```python
from build123d import *

# Parameters (mm, degrees)
ENL_V_START             = -12
ENL_V_MAT_EXTRU_1_DEPTH = 12
ENL_V_START_2           = -3
ENL_V_MAT_EXTRU_2_DEPTH = 3
CHANFREIN1_SIZE         = 1
ENL_V_MAT_EXTRU_3_DEPTH = 3
ESQUISSE5_R             = 0.75
BOSS_EXTRU_1_DEPTH      = 0.5
CONG_1_R                = 0.5
ESQUISSE6_R             = 1.5
ENL_V_MAT_EXTRU_4_DEPTH = 5.5
CHANFREIN2_SIZE         = 1


with BuildPart() as part:
    # Esquisse1 → Révolution1 (revolve)
    with BuildSketch(Plane.XY):
        Polygon((0, 0), (0, 3), (17, 3), (17, 10), (20, 10), (20, 16), (60, 16), (60, 13.75), (100.5, 13.75), (100.5, 0), align=None)
    revolve(axis=Axis((100.5, 0, 0), (-1, 0, 0)))

    # Esquisse2 → Enlèv. mat.-Extru.1 (cut)
    with BuildSketch(Plane.ZY.offset(ENL_V_START)):
        with BuildLine():
            Line((-1.658312395, 2.5), (1.658312395, 2.5))
            ThreePointArc((1.658312395, 2.5), (0, 3), (-1.658312395, 2.5))
        make_face()
    extrude(amount=ENL_V_MAT_EXTRU_1_DEPTH, mode=Mode.SUBTRACT)

    # Esquisse3 → Enlèv. mat.-Extru.2 (cut)
    with BuildSketch(Plane.ZY.offset(-17).offset(ENL_V_START_2)):
        with BuildLine():
            ThreePointArc((-9, 4.358898944), (-10, 0), (-9, -4.358898944))
            Line((-9, -4.358898944), (-9, 4.358898944))
        make_face()
        with BuildLine():
            Line((9, 4.358898944), (9, -4.358898944))
            ThreePointArc((9, -4.358898944), (9.746794345, -2.236067977), (10, 0))
            ThreePointArc((10, 0), (9.746794345, 2.236067977), (9, 4.358898944))
        make_face()
    extrude(amount=ENL_V_MAT_EXTRU_2_DEPTH, mode=Mode.SUBTRACT)

    # Chanfrein1
    chanfrein1_edges = [part.edges().sort_by_distance(p)[0] for p in [
        (20, -16, 0),
    ]]
    chamfer(chanfrein1_edges, length=CHANFREIN1_SIZE)

    # Esquisse4 → Enlèv. mat.-Extru.3 (cut)
    with BuildSketch(Plane.ZY.offset(-20)):
        with BuildLine():
            Line((16, 1.5), (15, 1.5))
            ThreePointArc((15, 1.5), (13.5, 0), (15, -1.5))
            Line((15, -1.5), (16, -1.5))
            Line((16, -1.5), (16, 1.5))
        make_face()
        with BuildLine():
            Line((1.5, -16), (1.5, -15))
            ThreePointArc((1.5, -15), (0, -13.5), (-1.5, -15))
            Line((-1.5, -15), (-1.5, -16))
            Line((-1.5, -16), (1.5, -16))
        make_face()
        with BuildLine():
            Line((-16, -1.5), (-15, -1.5))
            ThreePointArc((-15, -1.5), (-13.5, 0), (-15, 1.5))
            Line((-15, 1.5), (-16, 1.5))
            Line((-16, 1.5), (-16, -1.5))
        make_face()
        with BuildLine():
            Line((-1.5, 16), (-1.5, 15))
            ThreePointArc((-1.5, 15), (0, 13.5), (1.5, 15))
            Line((1.5, 15), (1.5, 16))
            Line((1.5, 16), (-1.5, 16))
        make_face()
    extrude(amount=-ENL_V_MAT_EXTRU_3_DEPTH, mode=Mode.SUBTRACT)

    # Esquisse5 → Boss.-Extru.1 (add)
    with BuildSketch(Plane.ZY.offset(-23)):
        with Locations(Location((0, 15, 0), (0, 0, 270))):
            Circle(ESQUISSE5_R)
        with Locations(Location((15, 0, 0), (0, 0, 270))):
            Circle(ESQUISSE5_R)
        with Locations(Location((0, -15, 0), (0, 0, 270))):
            Circle(ESQUISSE5_R)
        with Locations(Location((-15, 0, 0), (0, 0, 270))):
            Circle(ESQUISSE5_R)
    extrude(amount=BOSS_EXTRU_1_DEPTH)

    # Congé1
    cong_1_edges = [part.edges().sort_by_distance(p)[0] for p in [
        (22.5, 15.75, 0),
        (22.5, 0.75, 15),
        (22.5, -14.25, 0),
        (22.5, 0.75, -15),
    ]]
    fillet(cong_1_edges, radius=CONG_1_R - 0.0001)  # a hair under: the kernel refuses the full size

    # Esquisse6 → Enlèv. mat.-Extru.4 (cut)
    with BuildSketch(Plane.ZY.offset(-20)):
        with Locations(Location((9.192388155, 9.192388155, 0), (0, 0, 270))):
            Circle(ESQUISSE6_R)
        with Locations(Location((9.192388155, -9.192388155, 0), (0, 0, 270))):
            Circle(ESQUISSE6_R)
        with Locations(Location((-9.192388155, -9.192388155, 0), (0, 0, 270))):
            Circle(ESQUISSE6_R)
        with Locations(Location((-9.192388155, 9.192388155, 0), (0, 0, 270))):
            Circle(ESQUISSE6_R)
    extrude(amount=-ENL_V_MAT_EXTRU_4_DEPTH, mode=Mode.SUBTRACT)

    # Chanfrein2
    chanfrein2_edges = [part.edges().sort_by_distance(p)[0] for p in [
        (100.5, -13.75, 0),
    ]]
    chamfer(chanfrein2_edges, length=CHANFREIN2_SIZE)


solid = part.part
```
Geometry check sheet. Reference: the model listing, model coordinates, mm. A direction names the side the tool comes from. Round coordinates to 2 decimals unless told otherwise and drop trailing zeros. Order: outer loops, then holes, each group sorted by start corner. A loop starts at its lowest first (then second) coordinate and runs counter-clockwise, first axis right, second up. Notation, with made-up numbers: (25.5, -39.75) - (33.5, -39.75) arc R25 cw to (33.5, -21.75) - close; hole circle Ø6 at (51, 27.25). An arc over 180 degrees is marked (long way). Use a Markdown table: item, result. Add a question column.
1) Set-up check for faces 1 (the conical face through (20.174, 10.625, 10.833)), 2 (the flat face through (0, 0, 0)), 3 (the cylindrical face through (19, -10, 0)), 4 (the cylindrical face through (80.026, -2.981, 13.423)), 5 (the flat face through (17, 2.4, -2.1)): record each of +Z, -Z, +X, -X, +Y, -Y from which the full face is reachable in a straight line by a thin tool's end or side.
2) Thickness scan on line 1 along X through (y, z) = (1.5, -10); line 2 along Y through (x, z) = (63.5, 2.5); line 3 along X through (y, z) = (-2, 5). Record the ranges inside material, lowest first.
3) Gauge pin test, flat ends, axial feed: P1, Ø2.5, axis at y = -10, z = 9, coming from the -X side; P2, Ø1.8, axis at y = -9.19, z = -9.19, coming from the -X side; P3, Ø0.9, axis at x = 18, y = -0.5, coming from the +Z side; P4, Ø5.5, axis at y = 2.5, z = -2, coming from the -X side. Record the tip position at first contact, or that the pin passes through.
4) Section check A-A (x = 40). Record the cut outline in (y, z), then the cut area to 3 significant figures.
5) Mould release check, pull along Y, two halves, no side actions. Record for faces 6 (the flat face through (23, 0, -14)), 7 (the cylindrical face through (40.77, -3.47, 15.62)), 8 (the flat face through (19, 0, 9)), 9 (the cylindrical face through (21.5, 0, -13.5)): released by +Y, released by -Y, zero draft, split by the parting line, or undercut.
Established:
| question | item | result |
|---|---|---|
| 1 | face 1 | +Z, -X, +Y |
| 1 | face 2 | +Z, -Z, -X, +Y, -Y |
| 1 | face 3 | -X, -Y |
| 1 | face 4 | +X |
| 1 | face 5 | -X |
| 2 | line 1 | 20 to 100.5 |
| 2 | line 2 | -13.52 to 13.52 |
| 2 | line 3 | 17 to 100.5 |
| 3 | P1 | x = 20 |
| 3 | P2 | x = 25.5 |
| 3 | P3 | z = 9 |
| 3 | P4 | x = 0 |
| 4 | outline | circle Ø32 at (0, 0) |
| 4 | area | 804 mm2 |
| 5 | face 6 | undercut |
| 5 | face 7 | split by the parting line |
| 5 | face 8 | zero draft |
| 5 | face 9 | undercut |
